Work out the finished part from the listing and answer in its coordinate system (mm). A direction names the side the tool comes from. Round coordinates to 2 decimals unless told otherwise and drop trailing zeros. Order: outer loops, then holes, each group sorted by start corner. A loop starts at its lowest first (then second) coordinate and runs counter-clockwise, first axis right, second up. Notation, with made-up numbers: (84, 83) -> (116, 83) arc R13 ccw to (116, 92) -> close; hole circle Ø11 at (17, -34). An arc over 180 degrees is marked (long way). Use a Markdown table: item, result. Add a question column.
Item 1: A cutting plane is placed at A-A, the plane x = -3.5. Determine the outline of the cut face in (y, z) (1 decimal), plus the area to 3 significant figures.
Item 2: A tool of negligible diameter and unlimited length cuts with its end or side. For faces 1 (the flat face through (25, 0, 0)), 2 (the flat face through (0, 0, -6)), 3 (the cylindrical face through (-7.419, -1.382, 6.223)), from which of +Z, -Z, +X, -X, +Y, -Y can it reach the whole face along a straight path? Write none if from no direction.
Item 3: A cutting plane is placed at B-B, the plane x = 3.5. Determine the outline of the cut face in (y, z).
Item 4: Find the intervals of material crossed by L1, parallel to Y at x = -7.5, z = 0 (3 decimals); L2, parallel to X at y = 3.5, z = -2; L3, parallel to X at y = -6.75, z = 0, in increasing order. Write a range as [from, to].
Item 5: For a pull along Z with two mould halves and no side action, classify faces 4 (the flat face through (-6.584, 0, 0)), 5 (the flat face through (-8.23, 3, 6)), 6 (the conical face through (-0.13, -0.19, 8.72)) as +Z half, -Z half, draft (parallel to the pull), parting line (faces both ways), or undercut.
Item 6: Flat-ended cylindrical pins translate along their axes: P1, Ø1, axis at x = 4, y = 3.5, coming from the -Z side; P2, Ø6.5, axis at y = -0.5, z = -1, coming from the -X side; P3, Ø1, axis at x = 2, z = 2.5, coming from the -Y side. Find the tip coordinate at first contact, or state that the pin passes through.
Autodesk Inventor part; units mm, degrees
ref_plane "Work Plane1" through (3, 0, 0) normal (0, 0.5, 0.866) x (1, 0, 0)
ref_plane "YZ Plane" through (0, 0, 0) normal (1, 0, 0) x (0, 1, 0)
ref_plane "XZ Plane" through (0, 0, 0) normal (0, 1, 0) x (-1, 0, 0)
sketch "Sketch1" plane through (0, 0, 0) normal (0, 0, 1) x (1, 0, 0)
  line L0 (0, 5) -> (0, 0)
  line L1 (0, 0) -> (25, 0)
  line L2 (25, 0) -> (25, 5)
  line L3 (25, 5) -> (0, 5)
  line L4 (-5, 0) -> (30, 0)
  line L5 (0, -1) -> (0, 6)
  dimension "d0" = 10
  dimension "d1" = 25
revolve "Body" add sketch "Sketch1" angle 360 about axis through (0, 0, 0) along (1, 0, 0)
sketch "Sketch2" plane through (0, 0, 0) normal (1, 0, 0) x (0, 1, 0)
  line L0 (0, 9.815) -> (8.5, 4.9075)
  line L1 (8.5, 4.9075) -> (8.5, -4.9075)
  line L2 (8.5, -4.9075) -> (0, -9.815)
  line L3 (0, -9.815) -> (-8.5, -4.9075)
  line L4 (-8.5, -4.9075) -> (-8.5, 4.9075)
  line L5 (-8.5, 4.9075) -> (0, 9.815)
  line L6 (-11.9, 0) -> (11.9, 0)
  line L7 (0, -13.7409) -> (0, 13.7409)
  point P0 (0, 0)
  point P1 (0, 0)
  dimension "d2" = 17
extrude "Head" add sketch "Sketch2" against normal blind 8.23
sketch "Sketch3" plane through (-8.23, 0, 0) normal (-1, 0, 0) x (0, 1, 0)
  circle A0 centre (0, 0) radius 6.375
  point P0 (0, 0)
  dimension "d12" = 12.75
extrude "Indent1" cut sketch "Sketch3" against normal blind 1.646
sketch "Sketch4" plane through (0, 0, 0) normal (0, 0, 1) x (1, 0, 0)
  line L0 (-8.23, 9.815) -> (-8.23, 8.5)
  line L1 (-8.23, 8.5) -> (-7.4708, 9.815)
  line L2 (-7.4708, 9.815) -> (-8.23, 9.815)
  line L3 (0, 9.815) -> (0, 8.5)
  line L4 (0, 8.5) -> (-0.7592, 9.815)
  line L5 (-0.7592, 9.815) -> (0, 9.815)
  line L6 (0, 0) -> (-8.23, 0)
  line L7 (-8.23, 0) -> (-8.23, 8.5)
  line L8 (0, 0) -> (0, 8.5)
  line L9 (-9.876, 0) -> (1.646, 0)
  line L10 (-7.4708, 9.815) -> (-0.7592, 9.815) construction
  line L11 (0, -1.963) -> (0, 11.7779)
  dimension "d6" = 30
  dimension "d7" = 30
  dimension "d16" = 17
  dimension "d17" = 17
  dimension "d18" = 19.6299
revolve "Chamfer1" cut sketch "Sketch4" angle 360 about axis through (-10, 0, 0) along (1, 0, 0)
fillet "Fillet1" radius 0.4 1 edges at (0, -5, 0)
thread "Thread"
ref_plane "Work Plane1" through (3, 0, 0) normal (0, 0.5, 0.866) x (1, 0, 0)
equation "\"d0\" = GD"
equation "\"d1\" = NLG"
equation "\"d2\" = SW"
equation "\"d3\" = KOH"
equation "\"d12\" = 0.75 * SW0"
equation "\"d14\" = 0.2 * KOH"
equation "\"d6\" = ANG1"
equation "\"d7\" = ANG1"
equation "\"d16\" = SW0"
equation "\"d17\" = SW0"
equation "\"d18\" = 1.1547 * SW"
equation "\"d11\" = RR"
equation "\"d8\" = GEL"
equation "\"NLG\" = 25"
equation "\"KOH\" = 8.23"
equation "\"GD\" = NND"
equation "\"GEL\" = 22"
equation "\"SW\" = 17"
equation "\"SW0\" = SW"
equation "\"ANG1\" = 30deg"
equation "\"RR\" = 0.4"
equation "\"GUL\" = 0.61345 * PTC"
equation "\"SPD\" = NND - 1.2269 * PTC"
equation "\"GD1\" = THREADDIA - 1.2269 * PTC"
equation "\"SDH\" = 11.2"
equation "\"TOA\" = 30deg"
equation "\"FAWI\" = 45deg"
equation "\"PTC\" = 1.5"
equation "\"GAL\" = 0.61345 * PTC"
equation "\"SD\" = 0"
equation "\"SD2\" = SDH"
equation "\"E0\" = 1.155 * SW"
properties part number "AS 1427 - M10 x 25" material "Steel, Mild"
Reported:
| question | item | result |
|---|---|---|
| 1 | outline | (-8.5, -4.9) -> (0, -9.8) -> (8.5, -4.9) -> (8.5, 4.9) -> (0, 9.8) -> (-8.5, 4.9) -> close |
| 1 | area | 250 mm² |
| 2 | face 1 | +Z, -Z, +X, +Y, -Y |
| 2 | face 2 | +X |
| 2 | face 3 | -X |
| 3 | outline | circle Ø10 at (0, 0) |
| 4 | L1 | [-8.5, -6.375], [6.375, 8.5] |
| 4 | L2 | [-6.58, 25] |
| 4 | L3 | [-8.23, 0] |
| 5 | face 4 | undercut |
| 5 | face 5 | draft |
| 5 | face 6 | +Z half |
| 6 | P1 | z = -4 |
| 6 | P2 | x = -6.58 |
| 6 | P3 | y = -4.58 |
